Read the model definition and answer for the solid it produces. Units are mm, in the model's axes. A direction names the side the tool comes from. Give positions to 0.01 mm unless a question says otherwise; leave off trailing zeros. Order: outer loops, then holes, each group sorted by start corner. A loop starts at its lowest first (then second) coordinate and runs counter-clockwise, first axis right, second up.
```python
from build123d import *

# Parameters (mm, degrees)
SKETCH1_W                                = 88
SKETCH1_H                                = 65
BOSS_EXTRUDE2_DEPTH                      = 1.8
FILLET1_R                                = 10
F_12_2_12_2_DIAMETER_HOLE1_D             = 12.2
BOSS_EXTRUDE3_START                      = 10
BOSS_EXTRUDE3_DEPTH                      = 10
SKETCH5_W                                = 40
SKETCH5_H                                = 11.65
SKETCH5_W_2                              = 11.15
SKETCH5_H_2                              = 30
BOSS_EXTRUDE4_DEPTH                      = 10.5
SKETCH6_R                                = 2.55
CUT_EXTRUDE1_DEPTH                       = 5
CUT_EXTRUDE1_DRAFT                       = -2
CUT_EXTRUDE1_PROFILE_2_DEPTH             = 5
CUT_EXTRUDE1_PROFILE_2_DRAFT             = -2
CUT_EXTRUDE1_PROFILE_3_DEPTH             = 5
CUT_EXTRUDE1_PROFILE_3_DRAFT             = -2
CUT_EXTRUDE1_PROFILE_4_DEPTH             = 5
CUT_EXTRUDE1_PROFILE_4_DRAFT             = -2
CUT_EXTRUDE1_PROFILE_5_DEPTH             = 5
CUT_EXTRUDE1_PROFILE_5_DRAFT             = -2
CUT_EXTRUDE1_PROFILE_6_DEPTH             = 5
CUT_EXTRUDE1_PROFILE_6_DRAFT             = -2
CUT_EXTRUDE1_PROFILE_7_DEPTH             = 5
CUT_EXTRUDE1_PROFILE_7_DRAFT             = -2
SKETCH7_R                                = 2.5
CUT_EXTRUDE2_DEPTH                       = 111.092188642
BOSS_EXTRUDE5_DEPTH                      = 12
MIRROR1_AT_THE_SECOND_PLANE_COPY_1_DEPTH = 12


with BuildPart() as part:
    # Sketch1 → Boss-Extrude2 (new body)
    with BuildSketch(Plane(origin=(0, 0, 0), x_dir=(1, 0, 0), z_dir=(0, 1, 0))):
        with Locations((44, 32.5)):
            Rectangle(SKETCH1_W, SKETCH1_H)
    extrude(amount=BOSS_EXTRUDE2_DEPTH)

    # Fillet1
    fillet1_edges = [part.edges().sort_by_distance(p)[0] for p in [
        (0, 0.9, -65),
        (88, 0.9, -65),
        (88, 0.9, 0),
        (0, 0.9, 0),
    ]]
    fillet(fillet1_edges, radius=FILLET1_R)

    # Ø12.2 (12.2) Diameter Hole1 (through all)
    with Locations(Plane(origin=(0, 1.8, 0), x_dir=(1, 0, 0), z_dir=(0, 1, 0))):
        with Locations((7.805, 55.36), (80.195, 55.36), (7.805, 9.64), (80.195, 9.64)):
            Hole(F_12_2_12_2_DIAMETER_HOLE1_D / 2)

    # Sketch4 → Boss-Extrude3 (add)
    with BuildSketch(Plane(origin=(0, 1.8, 0), x_dir=(1, 0, 0), z_dir=(0, 1, 0)).offset(BOSS_EXTRUDE3_START)):
        with BuildLine():
            Line((78, 65), (10, 65))
            ThreePointArc((10, 65), (2.928932188, 62.071067812), (0, 55))
            Line((0, 55), (0, 10))
            ThreePointArc((0, 10), (2.928932188, 2.928932188), (10, 0))
            Line((10, 0), (78, 0))
            ThreePointArc((78, 0), (85.071067812, 2.928932188), (88, 10))
            Line((88, 10), (88, 55))
            ThreePointArc((88, 55), (85.071067812, 62.071067812), (78, 65))
        make_face()
        with BuildLine():
            Line((78, 63.4), (10, 63.4))
            ThreePointArc((10, 63.4), (4.060303038, 60.939696962), (1.6, 55))
            Line((1.6, 55), (1.6, 10))
            ThreePointArc((1.6, 10), (4.060303038, 4.060303038), (10, 1.6))
            Line((10, 1.6), (78, 1.6))
            ThreePointArc((78, 1.6), (83.939696962, 4.060303038), (86.4, 10))
            Line((86.4, 10), (86.4, 55))
            ThreePointArc((86.4, 55), (83.939696962, 60.939696962), (78, 63.4))
        make_face(mode=Mode.SUBTRACT)
    extrude(amount=-BOSS_EXTRUDE3_DEPTH)

    # Sketch5 → Boss-Extrude4 (add)
    with BuildSketch(Plane(origin=(0, 1.8, 0), x_dir=(1, 0, 0), z_dir=(0, 1, 0))):
        with Locations((44, 57.575)):
            Rectangle(SKETCH5_W, SKETCH5_H)
        with Locations((44, 7.425)):
            Rectangle(SKETCH5_W, SKETCH5_H)
        with Locations((80.825, 32.5)):
            Rectangle(SKETCH5_W_2, SKETCH5_H_2)
        with Locations((7.175, 32.5)):
            Rectangle(SKETCH5_W_2, SKETCH5_H_2)
    extrude(amount=BOSS_EXTRUDE4_DEPTH)


with BuildPart() as cut_extrude1_tool:
    # Sketch6 → Cut-Extrude1 (with draft: the straight prism first)
    with BuildSketch(Plane(origin=(0, 12.3, 0), x_dir=(1, 0, 0), z_dir=(0, 1, 0))):
        with Locations((60, 56.9)):
            Circle(SKETCH6_R)
    extrude(amount=-CUT_EXTRUDE1_DEPTH)
    # Cut-Extrude1: the draft: its side faces are tilted about the plane it starts from
    cut_extrude1_sides = [cut_extrude1_tool.faces().sort_by_distance(p)[0] for p in [
        (57.45, 9.8, -56.9),
    ]]
    draft(cut_extrude1_sides, Plane(origin=(0, 12.3, 0), x_dir=(1, 0, 0), z_dir=(0, 1, 0)), CUT_EXTRUDE1_DRAFT)


with BuildPart() as part_1:
    add(part.part)

    # Cut-Extrude1: cut by cut_extrude1_tool
    add(cut_extrude1_tool.part, mode=Mode.SUBTRACT)


with BuildPart() as cut_extrude1_profile_2_tool:
    # Sketch6 → Cut-Extrude1 profile 2 (with draft: the straight prism first)
    with BuildSketch(Plane(origin=(0, 12.3, 0), x_dir=(1, 0, 0), z_dir=(0, 1, 0))):
        with Locations((28, 56.9)):
            Circle(SKETCH6_R)
    extrude(amount=-CUT_EXTRUDE1_PROFILE_2_DEPTH)
    # Cut-Extrude1 profile 2: the draft: its side faces are tilted about the plane it starts from
    cut_extrude1_profile_2_sides = [cut_extrude1_profile_2_tool.faces().sort_by_distance(p)[0] for p in [
        (25.45, 9.8, -56.9),
    ]]
    draft(cut_extrude1_profile_2_sides, Plane(origin=(0, 12.3, 0), x_dir=(1, 0, 0), z_dir=(0, 1, 0)), CUT_EXTRUDE1_PROFILE_2_DRAFT)


with BuildPart() as part_2:
    add(part_1.part)

    # Cut-Extrude1 profile 2: cut by cut_extrude1_profile_2_tool
    add(cut_extrude1_profile_2_tool.part, mode=Mode.SUBTRACT)


with BuildPart() as cut_extrude1_profile_3_tool:
    # Sketch6 → Cut-Extrude1 profile 3 (with draft: the straight prism first)
    with BuildSketch(Plane(origin=(0, 12.3, 0), x_dir=(1, 0, 0), z_dir=(0, 1, 0))):
        with Locations((4.6, 43.5)):
            Circle(SKETCH6_R)
    extrude(amount=-CUT_EXTRUDE1_PROFILE_3_DEPTH)
    # Cut-Extrude1 profile 3: the draft: its side faces are tilted about the plane it starts from
    cut_extrude1_profile_3_sides = [cut_extrude1_profile_3_tool.faces().sort_by_distance(p)[0] for p in [
        (2.05, 9.8, -43.5),
    ]]
    draft(cut_extrude1_profile_3_sides, Plane(origin=(0, 12.3, 0), x_dir=(1, 0, 0), z_dir=(0, 1, 0)), CUT_EXTRUDE1_PROFILE_3_DRAFT)


with BuildPart() as part_3:
    add(part_2.part)

    # Cut-Extrude1 profile 3: cut by cut_extrude1_profile_3_tool
    add(cut_extrude1_profile_3_tool.part, mode=Mode.SUBTRACT)


with BuildPart() as cut_extrude1_profile_4_tool:
    # Sketch6 → Cut-Extrude1 profile 4 (with draft: the straight prism first)
    with BuildSketch(Plane(origin=(0, 12.3, 0), x_dir=(1, 0, 0), z_dir=(0, 1, 0))):
        with Locations((4.6, 27.106324955)):
            Circle(SKETCH6_R)
    extrude(amount=-CUT_EXTRUDE1_PROFILE_4_DEPTH)
    # Cut-Extrude1 profile 4: the draft: its side faces are tilted about the plane it starts from
    cut_extrude1_profile_4_sides = [cut_extrude1_profile_4_tool.faces().sort_by_distance(p)[0] for p in [
        (2.05, 9.8, -27.106324955),
    ]]
    draft(cut_extrude1_profile_4_sides, Plane(origin=(0, 12.3, 0), x_dir=(1, 0, 0), z_dir=(0, 1, 0)), CUT_EXTRUDE1_PROFILE_4_DRAFT)


with BuildPart() as part_4:
    add(part_3.part)

    # Cut-Extrude1 profile 4: cut by cut_extrude1_profile_4_tool
    add(cut_extrude1_profile_4_tool.part, mode=Mode.SUBTRACT)


with BuildPart() as cut_extrude1_profile_5_tool:
    # Sketch6 → Cut-Extrude1 profile 5 (with draft: the straight prism first)
    with BuildSketch(Plane(origin=(0, 12.3, 0), x_dir=(1, 0, 0), z_dir=(0, 1, 0))):
        with Locations((83.4, 21.5)):
            Circle(SKETCH6_R)
    extrude(amount=-CUT_EXTRUDE1_PROFILE_5_DEPTH)
    # Cut-Extrude1 profile 5: the draft: its side faces are tilted about the plane it starts from
    cut_extrude1_profile_5_sides = [cut_extrude1_profile_5_tool.faces().sort_by_distance(p)[0] for p in [
        (80.85, 9.8, -21.5),
    ]]
    draft(cut_extrude1_profile_5_sides, Plane(origin=(0, 12.3, 0), x_dir=(1, 0, 0), z_dir=(0, 1, 0)), CUT_EXTRUDE1_PROFILE_5_DRAFT)


with BuildPart() as part_5:
    add(part_4.part)

    # Cut-Extrude1 profile 5: cut by cut_extrude1_profile_5_tool
    add(cut_extrude1_profile_5_tool.part, mode=Mode.SUBTRACT)


with BuildPart() as cut_extrude1_profile_6_tool:
    # Sketch6 → Cut-Extrude1 profile 6 (with draft: the straight prism first)
    with BuildSketch(Plane(origin=(0, 12.3, 0), x_dir=(1, 0, 0), z_dir=(0, 1, 0))):
        with Locations((83.4, 43.5)):
            Circle(SKETCH6_R)
    extrude(amount=-CUT_EXTRUDE1_PROFILE_6_DEPTH)
    # Cut-Extrude1 profile 6: the draft: its side faces are tilted about the plane it starts from
    cut_extrude1_profile_6_sides = [cut_extrude1_profile_6_tool.faces().sort_by_distance(p)[0] for p in [
        (80.85, 9.8, -43.5),
    ]]
    draft(cut_extrude1_profile_6_sides, Plane(origin=(0, 12.3, 0), x_dir=(1, 0, 0), z_dir=(0, 1, 0)), CUT_EXTRUDE1_PROFILE_6_DRAFT)


with BuildPart() as part_6:
    add(part_5.part)

    # Cut-Extrude1 profile 6: cut by cut_extrude1_profile_6_tool
    add(cut_extrude1_profile_6_tool.part, mode=Mode.SUBTRACT)


with BuildPart() as cut_extrude1_profile_7_tool:
    # Sketch6 → Cut-Extrude1 profile 7 (with draft: the straight prism first)
    with BuildSketch(Plane(origin=(0, 12.3, 0), x_dir=(1, 0, 0), z_dir=(0, 1, 0))):
        with Locations((44, 8.1)):
            Circle(SKETCH6_R)
    extrude(amount=-CUT_EXTRUDE1_PROFILE_7_DEPTH)
    # Cut-Extrude1 profile 7: the draft: its side faces are tilted about the plane it starts from
    cut_extrude1_profile_7_sides = [cut_extrude1_profile_7_tool.faces().sort_by_distance(p)[0] for p in [
        (41.45, 9.8, -8.1),
    ]]
    draft(cut_extrude1_profile_7_sides, Plane(origin=(0, 12.3, 0), x_dir=(1, 0, 0), z_dir=(0, 1, 0)), CUT_EXTRUDE1_PROFILE_7_DRAFT)


with BuildPart() as part_7:
    add(part_6.part)

    # Cut-Extrude1 profile 7: cut by cut_extrude1_profile_7_tool
    add(cut_extrude1_profile_7_tool.part, mode=Mode.SUBTRACT)

    # Sketch7 → Cut-Extrude2 (cut, through all)
    with BuildSketch(Plane.XZ):
        with Locations(Location((44, -50, 0), (0, 0, 270))):
            Circle(SKETCH7_R)
    extrude(amount=-CUT_EXTRUDE2_DEPTH, mode=Mode.SUBTRACT)

    # Sketch8 → Boss-Extrude5 (add)
    with BuildSketch(Plane.ZY.offset(-24)):
        Polygon((-1.6, 9.799528107), (-1.6, 11.8), (-2.6, 10.821488431), align=None)
    boss_extrude5 = extrude(amount=BOSS_EXTRUDE5_DEPTH)

    # Mirror1: Boss-Extrude5 across plane
    add(boss_extrude5.mirror(Plane.XY.offset(-32.5)))

    # Mirror1 at the second plane: Boss-Extrude5 across plane
    add(boss_extrude5.mirror(Plane.ZY.offset(-44)))

    # Mirror1 at the second plane copy 1 sketc → Mirror1 at the second plane copy 1 (add)
    with BuildSketch(Plane(origin=(64, 0, -65), x_dir=(0, 0, -1), z_dir=(1, 0, 0))):
        Polygon((-1.6, 9.799528107), (-1.6, 11.8), (-2.6, 10.821488431), align=None)
    extrude(amount=MIRROR1_AT_THE_SECOND_PLANE_COPY_1_DEPTH)


solid = part_7.part
```
1) The part is cut by section B-B on z = -21.5. Determine the outline of the cut face in (x, y).
Final values:
outline: (0, 0) - (88, 0) - (88, 11.8) - (86.4, 11.8) - (86.4, 12.3) - (85.95, 12.3) - (85.78, 7.3) - (81.02, 7.3) - (80.85, 12.3) - (75.25, 12.3) - (75.25, 1.8) - (12.75, 1.8) - (12.75, 12.3) - (1.6, 12.3) - (1.6, 11.8) - (0, 11.8) - close
2) Consider L1, parallel to X at y = 1.35, z = -55.36 (3 decimals); L2, parallel to Z at x = 12, y = 2.75; L3, parallel to X at y = 6.25, z = -46.5. Determine where each line is inside the solid, lowest interval first.
Final values:
L1: x = 0.006 to 1.705, 13.905 to 74.095, 86.295 to 87.994
L2: z = -65 to -63.4, -47.5 to -17.5, -1.6 to 0
L3: x = 0 to 12.75, 75.25 to 88
3) A tool of negligible diameter and unlimited length cuts with its end or side. For faces 1 (the face through (1.6, 7, -14)), 2 (the face through (17, 6, -1.6)), 3 (the face through (12.301, 0.887, -13.763)), from which of +Z, -Z, +X, -X, +Y, -Y can it reach the whole face along a straight path? Write none if from no direction.
Final values:
face 1: +Y
face 2: none
face 3: +Y, -Y
4) The part is cut by section D-D on z = -50.5. Determine the outline of the cut face in (x, y), and give its area (3 significant figures).
Final values:
outline: (0, 0) - (4.12, 0) - (4.12, 1.8) - (1.6, 1.8) - (1.6, 11.8) - (0, 11.8) - close; (11.49, 0) - (41.55, 0) - (41.55, 1.8) - (11.49, 1.8) - close; (46.45, 0) - (76.51, 0) - (76.51, 1.8) - (46.45, 1.8) - close; (83.88, 0) - (88, 0) - (88, 11.8) - (86.4, 11.8) - (86.4, 1.8) - (83.88, 1.8) - close
area: 155 mm2
5) The part is cut by section C-C on x = 32. Determine the outline of the cut face in (y, z).
Final values:
outline: (0, -65) - (11.8, -65) - (11.8, -63.4) - (12.3, -63.4) - (12.3, -51.75) - (1.8, -51.75) - (1.8, -13.25) - (12.3, -13.25) - (12.3, -1.6) - (11.8, -1.6) - (11.8, 0) - (0, 0) - close
6) Given pin 1 (7.5 mm diameter, centred on x = 7.805, z = -9.64, fed in from +Y); pin 2 (1.4 mm diameter, centred on x = 84, z = -44.5, fed in from +Y); pin 3 (1 mm diameter, centred on x = 58, z = -15.5, fed in from +Y); pin 4 (1.1 mm diameter, centred on y = 11, z = -62.5, fed in from -X), each flat-ended and moving along its own axis, determine where each tip first touches the part or whether it passes through.
Final values:
pin 1: passes through
pin 2: stops at y = 7.3
pin 3: stops at y = 1.8
pin 4: stops at x = 2.81
7) For a pull along X with two mould halves and no side action, classify faces 4 (the face through (44, 12.3, -58)), 5 (the face through (75.25, 7, -32)) as released by +X, released by -X, zero draft, split by the parting line, or undercut.
Final values:
face 4: zero draft
face 5: undercut
